from build123d import *

# Parameters (mm, degrees)
SKETCH_1_W      = 710
SKETCH_1_H      = 300
EXTRUDE_1_DEPTH = 11.5
SKETCH_3_W      = 710
SKETCH_3_H      = 11.5
EXTRUDE_2_DEPTH = 89


with BuildPart() as part:
    # 草图1 → 凸台-拉伸1 (new body)
    with BuildSketch(Plane.XY):
        Rectangle(SKETCH_1_W, SKETCH_1_H)
    extrude(amount=EXTRUDE_1_DEPTH)

    # 草图3 → 凸台-拉伸2 (add)
    with BuildSketch(Plane.XY.offset(11.5)):
        with Locations((0, 144.25)):
            Rectangle(SKETCH_3_W, SKETCH_3_H)
    extrude_2 = extrude(amount=EXTRUDE_2_DEPTH)

    # 镜向1: 凸台-拉伸2 across plane
    add(extrude_2.mirror(Plane.ZX))


solid = part.part
The model under review builds one solid part; all positions refer to its coordinate system, in mm. A direction names the side the tool comes from. Give positions to 0.01 mm unless a question says otherwise; leave off trailing zeros. Order: outer loops, then holes, each group sorted by start corner. A loop starts at its lowest first (then second) coordinate and runs counter-clockwise, first axis right, second up. Notation, with made-up numbers: M 72.5,-39 L 105.5,-39 A32 ccw 105.5,-6 Z; hole C 60.25,62 d2. An arc over 180 degrees is marked long. One line per question, with ' | ' between items. Start each with the question number.
1) Consider section A-A, the plane z = 31. Give the boundary of the cut face in (x, y), then the cut area to 3 significant figures.
2) Mouldability with a two-part tool opening along Y and no side actions: class faces 1 (the face through (355, 1, 9)), 2 (the face through (-5, 150, 50)), 3 (the face through (-5, 138.5, 55)) as pulls with the +Y half, pulls with the -Y half, needs draft (parallel to the pull), parting line crosses it, or undercut.
3) For faces 4 (the face through (-355, 1, 9)), 5 (the face through (-5, -138.5, 55)), list the 3-axis set-ups (+Z, -Z, +X, -X, +Y, -Y) from which the entire face can be reached by the end or side of a thin tool; tool diameter is ignored.
4) Wall thickness on L1, parallel to Y at x = 229, z = 68.5; L2, parallel to Z at x = 67, y = 83: over which ranges is each line inside the solid? List them lowest first. Write a range as from..to.
5) Consider section C-C, the plane y = -8. Give the boundary of the cut face in (x, z), then the cut area to 4 significant figures.
6) Clearance check with a flat-ended pin moving along its axis: P1, Ø3, axis at x = -12, y = 54.5, coming from the +Z side. State where the tip first meets the part, or that it passes through.
7) Consider section B-B, the plane x = 230.5. Give the boundary of the cut face in (y, z), then the cut area to 3 significant figures.
Found:
1) outline: M -355,-150 L 355,-150 L 355,-138.5 L -355,-138.5 Z; M -355,138.5 L 355,138.5 L 355,150 L -355,150 Z | area: 16,300 mm²
2) face 1: needs draft | face 2: pulls with the +Y half | face 3: undercut
3) face 4: +Z, -Z, -X, +Y, -Y | face 5: +Z, +X, -X
4) L1: y = -150..-138.5, 138.5..150 | L2: z = 0..11.5
5) outline: M -355,0 L 355,0 L 355,11.5 L -355,11.5 Z | area: 8,165 mm²
6) P1: stops at z = 11.5
7) outline: M -150,0 L 150,0 L 150,100.5 L 138.5,100.5 L 138.5,11.5 L -138.5,11.5 L -138.5,100.5 L -150,100.5 Z | area: 5,500 mm²
